from build123d import *

# Parameters (mm, degrees)
CROQUIS1_R                 = 5
CROQUIS1_R_2               = 2.75
SALIENTE_EXTRUIR1_DEPTH    = 20
SALIENTE_EXTRUIR4_DEPTH    = 10
CROQUIS7_W                 = 42
CROQUIS7_H                 = 10
EXTRUIR_L_MINA1_DEPTH      = 20
CROQUIS8_W                 = 42.01139879
CROQUIS8_H                 = 12.793457143
SALIENTE_EXTRUIR6_DEPTH    = 26
REDONDEO1_R                = 2
REDONDEO2_R                = 1
CROQUIS9_W                 = 8.6
CROQUIS9_H                 = 15.7
CROQUIS9_W_2               = 5.6
CROQUIS9_H_2               = 12.6
SALIENTE_EXTRUIR7_DEPTH    = 6.4
CORTAR_EXTRUIR1_DEPTH      = 70.406702341
CORTAR_EXTRUIR1_DEPTH_BACK = 70.406702341
CROQUIS11_R                = 1.1
REDONDEO3_R                = 1
REDONDEO4_R                = 5
REDONDEO5_R                = 10


# Some blends are built 0.0001 mm under size
with BuildPart() as part:
    # Croquis1 → Saliente-Extruir1 (new body)
    with BuildSketch(Plane.XY):
        with BuildLine():
            Line((-5.025921035, -5.26753442), (-5.025921035, -8.26753442))
            ThreePointArc((-5.025921035, -8.26753442), (-0.025921035, -22.512532419), (4.974078965, -8.26753442))
            Line((4.974078965, -8.26753442), (4.974078965, -5.26753442))
            Line((4.974078965, -5.26753442), (5.974078965, -5.26753442))
            ThreePointArc((5.974078965, -5.26753442), (15.249563623, -2.724799651), (6.025921035, 0))
            Line((6.025921035, 0), (5.025921035, 0))
            Line((5.025921035, 0), (-5.025921035, 0))
            Line((-5.025921035, 0), (-6.025921035, 0))
            ThreePointArc((-6.025921035, 0), (-15.276011655, -2.63376721), (-6.025921035, -5.26753442))
            Line((-6.025921035, -5.26753442), (-5.025921035, -5.26753442))
        make_face()
        with Locations((-0.025921035, -14.512532419)):
            Circle(CROQUIS1_R, mode=Mode.SUBTRACT)
        with Locations((-10.276011655, -2.63376721)):
            Circle(CROQUIS1_R_2, mode=Mode.SUBTRACT)
        with Locations(Location((10.249805759, -2.675592988, 0), (0, 0, 180))):
            Circle(CROQUIS1_R_2, mode=Mode.SUBTRACT)
    extrude(amount=SALIENTE_EXTRUIR1_DEPTH)

    # Croquis5 → Saliente-Extruir4 (add, symmetric)
    with BuildSketch(Plane(origin=(0, 0, 10), x_dir=(-1, 0, 0), z_dir=(0, 0, -1))):
        with BuildLine():
            Line((-7.974078965, -14.512532419), (-7.974078965, -32.592532419))
            Line((-7.974078965, -32.592532419), (8.025921035, -32.592532419))
            Line((8.025921035, -32.592532419), (8.025921035, -14.512532419))
            ThreePointArc((8.025921035, -14.512532419), (0.025921035, -22.512532419), (-7.974078965, -14.512532419))
        make_face()
    extrude(amount=SALIENTE_EXTRUIR4_DEPTH, both=True)

    # Croquis7 → Extruir-Lámina1 (add)
    with BuildSketch(Plane.XY.offset(20)):
        with Locations((-0.025921035, -27.592532419)):
            Rectangle(CROQUIS7_W, CROQUIS7_H)
    extrude(amount=-EXTRUIR_L_MINA1_DEPTH)

    # Croquis8 → Saliente-Extruir6 (add, symmetric)
    with BuildSketch(Plane.XY.offset(20)):
        with Locations((-0.02022164, -38.989260991)):
            Rectangle(CROQUIS8_W, CROQUIS8_H)
    extrude(amount=SALIENTE_EXTRUIR6_DEPTH, both=True)

    # Redondeo1
    # the kernel refuses this fillet: 2 mm, written as the material it adds along each edge
    with BuildSketch(Plane(origin=(-5.025921035, -8.26753442, 0), x_dir=(0, 1, 0), z_dir=(0, 0, 1))) as redondeo1_piece_1:
        with BuildLine():
            CenterArc((0.89643043, 2), REDONDEO1_R, 224.427004001, 45.572995999)
            Line((-0.531855256, 0.6), (-0.560420969, 0.572))
            ThreePointArc((-0.560420969, 0.572), (-0.288339065, 0.280133933), (-0.03122499, -0.025))
            Line((-0.03122499, -0.025), (0, -0.04))
            Line((0, -0.04), (0.89643043, -0.04))
            Line((0.89643043, -0.04), (0.89643043, 0))
        make_face()
    extrude(amount=20)
    with BuildSketch(Plane(origin=(4.974078965, -8.26753442, 0), x_dir=(0.7483239866610061, -0.6633334086172491, 0), z_dir=(0, 0, 1))) as redondeo1_piece_2:
        with BuildLine():
            CenterArc((0.902015721, 1.99748721), REDONDEO1_R, 221.554595727, 45.572995999)
            Line((-0.594632253, 0.670820393), (-0.624565212, 0.644287057))
            Line((-0.624565212, 0.644287057), (-0.029932959, -0.026533336))
            Line((-0.029932959, -0.026533336), (0.002004479, -0.039949744))
            ThreePointArc((0.002004479, -0.039949744), (0.400895876, -0.029948842), (0.799787272, -0.039949744))
            Line((0.799787272, -0.039949744), (0.801791752, 0))
        make_face()
    extrude(amount=20)
    with BuildSketch(Plane(origin=(-5.025921035, -5.26753442, 0), x_dir=(-1, 0, 0), z_dir=(0, 0, 1))) as redondeo1_piece_3:
        with BuildLine():
            CenterArc((2, 1.732050808), REDONDEO1_R, 180, 60)
            Line((0, 1.732050808), (-0.04, 1.732050808))
            Line((-0.04, 1.732050808), (-0.04, 0))
            Line((-0.04, 0), (0, -0.04))
            ThreePointArc((0, -0.04), (0.5, -0.04), (0.98, -0.034641016))
            Line((0.98, -0.034641016), (1, 0))
        make_face()
    extrude(amount=20)
    with BuildSketch(Plane(origin=(4.974078965, -5.26753442, 0), x_dir=(0, -1, 0), z_dir=(0, 0, 1))) as redondeo1_piece_4:
        with BuildLine():
            CenterArc((1.732050808, 2), REDONDEO1_R, 210, 60)
            Line((0, 1), (-0.034641016, 0.98))
            ThreePointArc((-0.034641016, 0.98), (-0.04, 0.5), (-0.04, 0))
            Line((-0.04, 0), (0, -0.04))
            Line((0, -0.04), (1.732050808, -0.04))
            Line((1.732050808, -0.04), (1.732050808, 0))
        make_face()
    extrude(amount=20)

    # Redondeo2
    redondeo2_edges = [part.edges().sort_by_distance(p)[0] for p in [
        (-6.025921035, -5.26753442, 10),
        (5.974078965, -5.26753442, 10),
    ]]
    fillet(redondeo2_edges, radius=REDONDEO2_R)

    # Croquis9 → Saliente-Extruir7 (add)
    with BuildSketch(Plane.XY.offset(20)):
        with Locations((0, 7.85)):
            Rectangle(CROQUIS9_W, CROQUIS9_H)
        with Locations((0.05, 7.85)):
            Rectangle(CROQUIS9_W_2, CROQUIS9_H_2, mode=Mode.SUBTRACT)
    extrude(amount=-SALIENTE_EXTRUIR7_DEPTH)

    # Croquis11 → Cortar-Extruir1 (cut, two sides: drawn at the far end of the back side and taken through both)
    with BuildSketch(Plane(origin=(4.3, 0, 0), x_dir=(0, 0, -1), z_dir=(1, 0, 0)).offset(-CORTAR_EXTRUIR1_DEPTH_BACK)):
        with Locations(Location((-16.899272709, 10.65, 0), (0, 0, 90))):
            Circle(CROQUIS11_R)
        with Locations(Location((-16.899272709, 4.15, 0), (0, 0, 90))):
            Circle(CROQUIS11_R)
    extrude(amount=CORTAR_EXTRUIR1_DEPTH + CORTAR_EXTRUIR1_DEPTH_BACK, mode=Mode.SUBTRACT)

    # Redondeo3
    redondeo3_edges = [part.edges().sort_by_distance(p)[0] for p in [
        (-5.162960517, 0, 20),
        (4.3, 7.85, 13.6),
        (4.3, 15.7, 16.8),
        (0, 0, 13.6),
        (4.3, 0, 16.8),
        (-4.3, 7.85, 13.6),
        (-4.3, 0, 16.8),
        (0, 15.7, 13.6),
        (-4.3, 15.7, 16.8),
        (4.3, 7.85, 20),
        (0, 15.7, 20),
        (-4.3, 7.85, 20),
        (5.162960517, 0, 20),
    ]]
    fillet(redondeo3_edges, radius=REDONDEO3_R)

    # Redondeo4
    redondeo4_edges = [part.edges().sort_by_distance(p)[0] for p in [
        (-8.025921035, -22.592532419, 10),
        (7.974078965, -22.592532419, 10),
    ]]
    fillet(redondeo4_edges, radius=REDONDEO4_R)

    # Redondeo5
    redondeo5_edges = [part.edges().sort_by_distance(p)[0] for p in [
        (-21.025921035, -22.592532419, 10),
        (20.974078965, -22.592532419, 10),
    ]]
    fillet(redondeo5_edges, radius=REDONDEO5_R - 0.0001)  # a hair under: the kernel refuses the full size


solid = part.part
Design review of the part built by this model. Coordinates are the model's own, in mm. A direction names the side the tool comes from. Give positions to 0.01 mm unless a question says otherwise; leave off trailing zeros. Order: outer loops, then holes, each group sorted by start corner. A loop starts at its lowest first (then second) coordinate and runs counter-clockwise, first axis right, second up. Notation, with made-up numbers: (6.25, 12) - (46.25, 12) arc R18 ccw to (46.25, 16) - close; hole circle Ø5 at (59.25, -30.75). An arc over 180 degrees is marked (long way). Write item = value, one per line. Start each with the question number.
Q1. We need section A-A on y = 4.15. State the section outline as (x, z) points, plus the area to 3 significant figures.
Q2. We need section C-C on y = -12. State the section outline as (x, z) points.
Q3. To check wall thickness, follow L1, parallel to X at y = -1, z = 9; L2, parallel to Z at x = 3.25, y = 4.15; L3, parallel to Y at x = 12.5, z = -1.5. State the ranges of each line that lie inside material, in increasing order. Write a range as from..to.
Q4. We need section B-B on z = 30.5. State the section outline as (x, y) points.
Q5. Clearance check with flat-ended pins moving along their axes: pin 1 Ø1.3 at (y, z) = (9, 16.5) entering from -X; pin 2 Ø8 at (x, y) = (-0.03, -14.51) entering from +Z; pin 3 Ø6 at (x, y) = (15.5, -2) entering from +Z; pin 4 Ø7 at (y, z) = (6.5, 15) entering from +X. State where each tip first meets the part, or that it passes through.
Q6. Tool access review of faces 4 (the face through (0, 1.55, 17)), 5 (the face through (-9.229, -20.846, 10.14)), 6 (the face through (0, -23, 0)): name each direction out of +Z, -Z, +X, -X, +Y, -Y from which nothing blocks a thin tool from reaching the whole face with its end or side.
Q7. We need section D-D on z = 6. State how many separate pieces and enclosed holes the cut face has, plus the area to 3 significant figures.
Q8. Mouldability with a two-part tool opening along Y and no side actions: class faces 1 (the face through (-4.3, 8, 17)), 2 (the face through (15.167, -1.768, 9.86)), 3 (the face through (0, -45.386, 20)) as released by +Y, released by -Y, zero draft, split by the parting line, or undercut.
Working result:
q1.outline = (-4.3, 14.6) arc R1 ccw to (-3.3, 13.6) - (-2.75, 13.6) - (-2.75, 15.8) - (-4.3, 15.8) - close; (-4.3, 18) - (-2.75, 18) - (-2.75, 20) - (-3.3, 20) arc R1 ccw to (-4.3, 19) - close; (2.85, 13.6) - (3.3, 13.6) arc R1 ccw to (4.3, 14.6) - (4.3, 15.8) - (2.85, 15.8) - close; (2.85, 18) - (4.3, 18) - (4.3, 19) arc R1 ccw to (3.3, 20) - (2.85, 20) - close
q1.area = 11.7 mm²
q2.outline = (-7.62, 0) - (-4.35, 0) - (-4.35, 20) - (-7.62, 20) - close; (4.3, 0) - (7.57, 0) - (7.57, 20) - (4.3, 20) - close
q3.L1 = -15..-12.49, -8.06..8.07, 12.43..14.96
q3.L2 = 13.6..15.8, 18..20
q3.L3 = -45.39..-32.59
q4.outline = (-21.03, -45.39) - (20.99, -45.39) - (20.99, -32.59) - (-21.03, -32.59) - close
q5.pin_1 = -4.3
q5.pin_2 = through
q5.pin_3 = 20
q5.pin_4 = 4.3
q6.face_4 = +Z, -Z
q6.face_5 = +Z, -Z, -X
q6.face_6 = -Z, +X, -X, +Y
q7.separate_pieces = 1
q7.enclosed_holes = 3
q7.area = 1,270 mm²
q8.face_1 = zero draft
q8.face_2 = undercut
q8.face_3 = released by -Y
